Part model, mm, in its own coordinate system. Face numbers are marked on the shaded views. A direction names the side the tool comes from. Round coordinates to 2 decimals unless told otherwise and drop trailing zeros. Loops run counter-clockwise (first coordinate to the right, second up) from the corner with the lowest first, then second, coordinate; pieces in that order, holes last. Notation, with made-up numbers: (19, -9) - (76, -9) arc R33 cw to (76, 20) - close; hole circle Ø11 at (64.25, 63). An arc over 180 degrees is marked (long way). Write each question's results on one line, items separated by ' | '. Start each with the question number.
(1) Tool access for the marked faces 1 and 2: list every direction of +Z, -Z, +X, -X, +Y, -Y with a clear straight run to the whole face (end or side of a thin tool).
(2) Cut at B-B, the plane z = -5.5. List the corners of the cut face in (x, y).
(3) Cut at D-D, the plane x = 24.5. List the corners of the cut face in (y, z).
(4) Cut at C-C, the plane y = -15.5. List the corners of the cut face in (x, z), then the cut area to 3 significant figures.
(5) Flat gauge pins, fed straight in: P1, Ø5.5, axis at x = 7.2, z = 0, coming from the -Y side; P2, Ø5, axis at x = 7.2, z = 0, coming from the +Y side. Where does each tip first touch, or does it go through?
(6) Cut at A-A, the plane x = 19.9. List the corners of the cut face in (y, z), then the cut area to 3 significant figures.
(7) Drill centre lines: L1, parallel to Z at x = 7.2, y = -9.25; L2, parallel to Z at x = 19.9, y = -1.4; L3, parallel to X at y = -28.5, z = 0.25. Where is each one in solid material? Low to high.
from build123d import *

# Parameters (mm, degrees)
SKETCH1_W                                      = 38.1
SKETCH1_H                                      = 85.1
BOSS_EXTRUDE1_DEPTH                            = 6.35
SKETCH2_W                                      = 25.4
SKETCH2_H                                      = 72.4
CUT_EXTRUDE1_DEPTH                             = 13.7
CBORE_FOR_6_SOCKET_HEAD_CAP_SCREW1_D           = 3.7973
CBORE_FOR_6_SOCKET_HEAD_CAP_SCREW1_CBORE_D     = 7.14502
CBORE_FOR_6_SOCKET_HEAD_CAP_SCREW1_CBORE_DEPTH = 3.7051996
CUT_EXTRUDE2_DEPTH                             = 13.7
CUT_EXTRUDE7_REACH                             = 14.7
F_4_40_TAPPED_HOLE1_D                          = 2.2606
F_4_40_TAPPED_HOLE1_DEPTH                      = 6.18
F_4_40_TAPPED_HOLE1_TIP                        = 0.679152758


with BuildPart() as part:
    # Sketch1 → Boss-Extrude1 (new body, symmetric)
    with BuildSketch(Plane.XY):
        with Locations((19.05, -42.55)):
            Rectangle(SKETCH1_W, SKETCH1_H)
    extrude(amount=BOSS_EXTRUDE1_DEPTH, both=True)

    # Sketch2 → Cut-Extrude1 (cut, through all)
    with BuildSketch(Plane.XY.offset(6.35)):
        with Locations((12.7, -48.9)):
            Rectangle(SKETCH2_W, SKETCH2_H)
    extrude(amount=-CUT_EXTRUDE1_DEPTH, mode=Mode.SUBTRACT)

    # CBORE for #6 Socket Head Cap Screw1 (through all)
    with Locations(Plane(origin=(0, 0, 0), x_dir=(-1, 0, 0), z_dir=(0, 1, 0))):
        with Locations((-7.2, 0), (-19.9, 0)):
            CounterBoreHole(CBORE_FOR_6_SOCKET_HEAD_CAP_SCREW1_D / 2, CBORE_FOR_6_SOCKET_HEAD_CAP_SCREW1_CBORE_D / 2, CBORE_FOR_6_SOCKET_HEAD_CAP_SCREW1_CBORE_DEPTH)

    # Sketch9 → Cut-Extrude2 (cut, through all)
    with BuildSketch(Plane.XY.offset(6.35)):
        with BuildLine():
            Line((25.4, -84.8), (36.685857157, -84.8))
            ThreePointArc((36.685857157, -84.8), (37.012701665, -85.021954446), (37.4, -85.1))
            Line((37.4, -85.1), (38.1, -85.1))
            Line((38.1, -85.1), (38.1, -88.1))
            Line((38.1, -88.1), (25.4, -88.1))
            Line((25.4, -88.1), (25.4, -84.8))
        make_face()
    extrude(amount=-CUT_EXTRUDE2_DEPTH, mode=Mode.SUBTRACT)

    # Sketch24 → Cut-Extrude7 (cut, up to next)
    with BuildSketch(Plane.XY.offset(6.35), mode=Mode.PRIVATE) as cut_extrude7_sk1:
        with BuildLine():
            Line((38.1, -85.1), (38, -85.1))
            ThreePointArc((38, -85.1), (37.296182614, -84.947443375), (36.71869987, -84.517157288))
            Line((36.71869987, -84.517157288), (37.001542582, -84.234314575))
            Line((37.001542582, -84.234314575), (25.4, -72.632771993))
            Line((25.4, -72.632771993), (22.894805483, -72.632771993))
            Line((22.894805483, -72.632771993), (22.894805483, -86.862285397))
            Line((22.894805483, -86.862285397), (38.1, -86.862285397))
            Line((38.1, -86.862285397), (38.1, -85.1))
        make_face()
    cut_extrude7_tool1 = extrude(cut_extrude7_sk1.sketch, amount=-CUT_EXTRUDE7_REACH, mode=Mode.PRIVATE) & part.part
    add(cut_extrude7_tool1.solids().sort_by_distance((28.474666, -81.452091, 6.35))[0], mode=Mode.SUBTRACT)

    # #4-40 Tapped Hole1
    with Locations(Plane(origin=(-19.288878517, -27.943893476, 153.694490084), x_dir=(0.707106781, -0.707106781, 0), z_dir=(-0.707106781, -0.707106781, 0))):
        with Locations((71.626370823, -150.519490084), (71.626370823, -156.869490084)):
            Hole(F_4_40_TAPPED_HOLE1_D / 2, depth=F_4_40_TAPPED_HOLE1_DEPTH)
            with Locations((0, 0, -(F_4_40_TAPPED_HOLE1_DEPTH + F_4_40_TAPPED_HOLE1_TIP / 2))):  # 118° drill point
                Cone(0, F_4_40_TAPPED_HOLE1_D / 2, F_4_40_TAPPED_HOLE1_TIP, mode=Mode.SUBTRACT)


solid = part.part
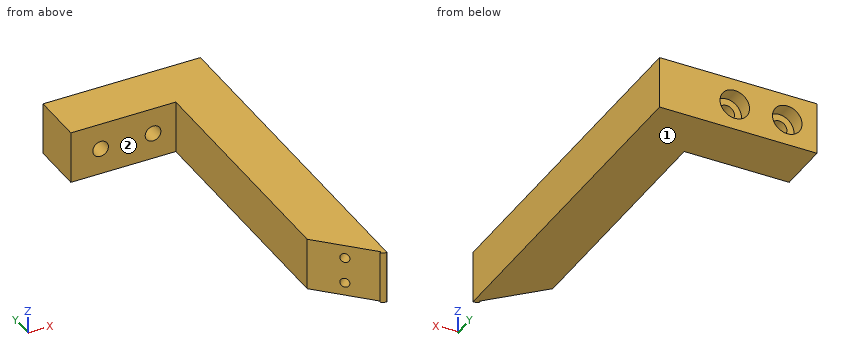
A:
1) face 1: -Z, +X, -X, +Y, -Y | face 2: +Z, -Z, -X, -Y
2) outline: (0, -12.7) - (25.4, -12.7) - (25.4, -72.63) - (37, -84.23) - (36.72, -84.52) arc R1.7 ccw to (38, -85.1) - (38.1, -85.1) - (38.1, 0) - (0, 0) - close
3) outline: (-12.7, -6.35) - (0, -6.35) - (0, 6.35) - (-12.7, 6.35) - close
4) outline: (25.4, -6.35) - (38.1, -6.35) - (38.1, 6.35) - (25.4, 6.35) - close | area: 161 mm2
5) P1: y = -12.7 | P2: y = -3.71
6) outline: (-12.7, -6.35) - (0, -6.35) - (0, -3.57) - (-3.71, -3.57) - (-3.71, -1.9) - (-12.7, -1.9) - close; (-12.7, 1.9) - (-3.71, 1.9) - (-3.71, 3.57) - (0, 3.57) - (0, 6.35) - (-12.7, 6.35) - close | area: 101 mm2
7) L1: -6.35 to -1.9, 1.9 to 6.35 | L2: -6.35 to -3.57, 3.57 to 6.35 | L3: 25.4 to 38.1
